Here's the drawing with two shaded views (mm, measured from the low corner). I have some questions. A direction names the side the tool comes from. Round coordinates to 2 decimals unless told otherwise and drop trailing zeros. Order: outer loops, then holes, each group sorted by start corner. A loop starts at its lowest first (then second) coordinate and runs counter-clockwise, first axis right, second up. Notation, with made-up numbers: (84, 72.25) - (100, 72.25) arc R19 ccw to (100, 89.25) - close; hole circle Ø10 at (39.5, 74). An arc over 180 degrees is marked (long way). Return JSON: item names as keys, results as strings. Group by question number.
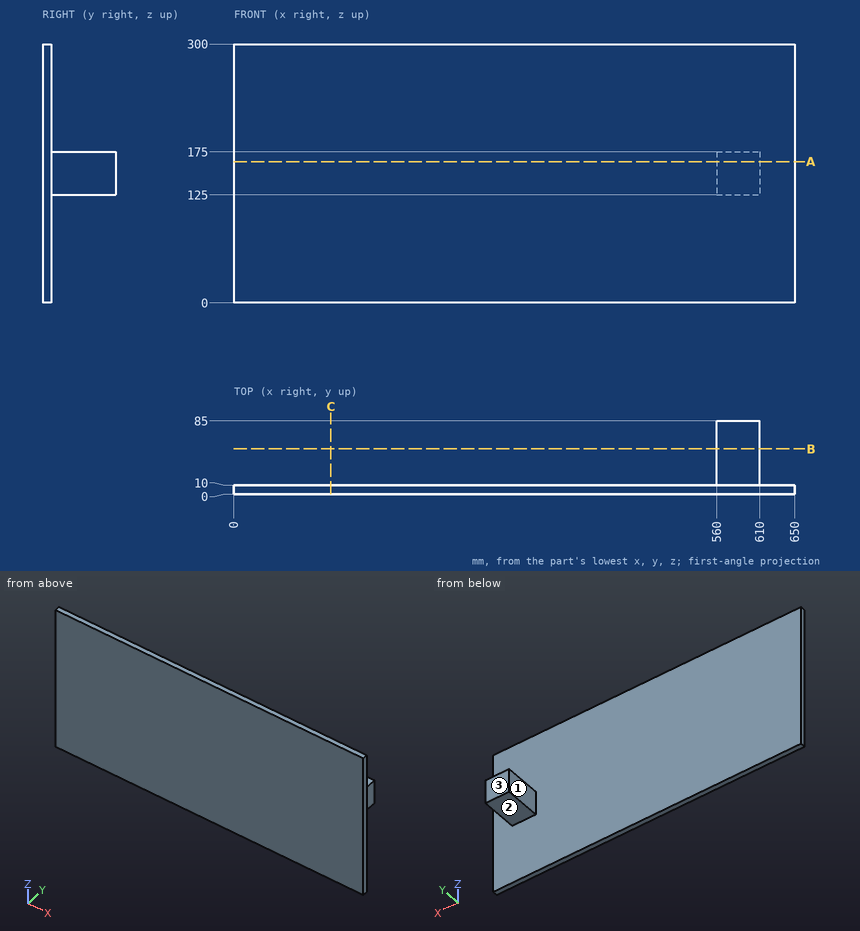
1) If I drill on line 1 along Y through (x, z) = (289.5, 98.5); line 2 along X through (y, z) = (74.5, 170); line 3 along Z through (x, y) = (566, 39), over which ranges is the centre line in solid material (lowest first)? Write a range as from..to.
2) I want a section at B-B, the plane y = 52.5. List the corners of the cut face in (x, z) for me, plus the area to 3 significant figures.
3) I want a section at A-A, the plane z = 163.5. List the corners of the cut face in (x, y) for me.
4) Will these pins go through, and if not, where does the flat tip stop? pin 1 (25 mm diameter, centred on y = 65.5, z = 158, fed in from -X); pin 2 (15 mm diameter, centred on x = 581, y = 48, fed in from +Z); pin 3 (25 mm diameter, centred on y = 31, z = 157, fed in from +X).
5) I want a section at C-C, the plane x = 112.5. List the corners of the cut face in (y, z) for me, plus the area to 3 significant figures.
6) For the marked faces 1, 2 and 3, which set-ups out of +Z, -Z, +X, -X, +Y, -Y let a thin tool reach every point of the face, with its end or its side?
Outcome:
{
 "1": {"line 1": "0..10", "line 2": "560..610", "line 3": "125..175"},
 "2": {"outline": "(560, 125) - (610, 125) - (610, 175) - (560, 175) - close", "area": "2,500 mm^2"},
 "3": {"outline": "(0, 0) - (650, 0) - (650, 10) - (610, 10) - (610, 85) - (560, 85) - (560, 10) - (0, 10) - close"},
 "4": {"pin 1": "x = 560", "pin 2": "z = 175", "pin 3": "x = 610"},
 "5": {"outline": "(0, 0) - (10, 0) - (10, 300) - (0, 300) - close", "area": "3,000 mm^2"},
 "6": {"face 1": "+Z, -Z, -X, +Y", "face 2": "-Z, +X, -X, +Y", "face 3": "+Z, -Z, +X, -X, +Y"}
}
